```python
from build123d import *

# Parameters (mm, degrees)
F0_R      = 55.0458583504
F1_DEPTH  = 4
F2_R      = 41.0058886934
F3_DEPTH  = 1
F4_R      = 11.9318178019
F5_DEPTH  = 2
F6_R      = 8.7944266384
F7_DEPTH  = 1
F8_R      = 5.553220806
F9_DEPTH  = 1
F11_DEPTH = 2
F13_DEPTH = 2


with BuildPart() as f1:
    # F0 (on Top) → F1 (new body)
    with BuildSketch(Plane.XY):
        Circle(F0_R)
    extrude(amount=F1_DEPTH)

    # F2 (on face) → F3 (join)
    with BuildSketch(Plane.XY.offset(4)):
        Circle(F2_R)
    extrude(amount=F3_DEPTH)

    # F4 (on face) → F5 (cut)
    with BuildSketch(Plane.XY.offset(5)):
        Circle(F4_R)
    extrude(amount=-F5_DEPTH, mode=Mode.SUBTRACT)

    # F6 (on face) → F7 (join)
    with BuildSketch(Plane.XY.offset(3)):
        Circle(F6_R)
    extrude(amount=F7_DEPTH)

    # F8 (on face) → F9 (join)
    with BuildSketch(Plane.XY.offset(4)):
        Circle(F8_R)
    extrude(amount=F9_DEPTH)

    # F10 (on face) → F11 (cut)
    with BuildSketch(Plane.XY.offset(5)):
        with BuildLine():
            Line((-11.5631810567, 2.9429780682), (-40.9001441028, 2.9429780682))
            ThreePointArc((-40.9001441028, 2.9429780682), (-41.0058886934, 0), (-40.9001441028, -2.9429780682))
            Line((-40.9001441028, -2.9429780682), (-11.5631810567, -2.9429780682))
            ThreePointArc((-11.5631810567, -2.9429780682), (-11.9318178019, 0), (-11.5631810567, 2.9429780682))
        make_face()
    extrude(amount=-F11_DEPTH, mode=Mode.SUBTRACT)

    # F12 (on face) → F13 (cut)
    with BuildSketch(Plane.XY.offset(5)):
        with BuildLine():
            Line((40.8989598294, 2.959390547), (11.5589914633, 2.959390547))
            ThreePointArc((11.5589914633, 2.959390547), (11.9318147961, 0.0084693883), (11.5631810567, -2.9429780682))
            Line((11.5631810567, -2.9429780682), (40.9001441028, -2.9429780682))
            ThreePointArc((40.9001441028, -2.9429780682), (41.005887868, 0.008227575), (40.8989598294, 2.959390547))
        make_face()
    extrude(amount=-F13_DEPTH, mode=Mode.SUBTRACT)


solid = f1.part
```
Can you work these out from the model? Positions are in its coordinate system, mm. A direction names the side the tool comes from. Give positions to 0.01 mm unless a question says otherwise; leave off trailing zeros. Order: outer loops, then holes, each group sorted by start corner. A loop starts at its lowest first (then second) coordinate and runs counter-clockwise, first axis right, second up. Notation, with made-up numbers: (52.5, 0) - (106.5, 0) arc R29 cw to (106.5, 33) - close; hole circle Ø2 at (69, 37). An arc over 180 degrees is marked (long way). Use a Markdown table: item, result. Add a question column.
Q1. If we mould it in two halves opening along X, with no side actions, what happens to faces 4 (the flat face through (0, 0, 5)), 5 (the flat face through (0, -6, 4)), 6 (the cylindrical face through (-0.22, -11.93, 4.01)), 7 (the cylindrical face through (0.852, 40.997, 4.493))? For each: released by +X, released by -X, zero draft, split by the parting line, or undercut.
Q2. On a 3-axis mill with a long thin cutter (end or side, diameter ignored), from which of +Z, -Z, +X, -X, +Y, -Y can I reach the whole of each face in a straight line? I mean faces 1 (the flat face through (-1, -22, 5)), 2 (the cylindrical face through (-0.86, -40.997, 4.493)), 3 (the cylindrical face through (-1.2, -5.42, 4.49)). Say none if no direction works.
Q3. If we section it at A-A on y = 0: Write out the boundary of the cut face in (x, z).
Q4. If we section it at C-C on z = 1.9: Write out the boundary of the cut face in (x, y).
Q5. If we section it at B-B on x = 0: Write out the boundary of the cut face in (y, z).
Q6. I'm going to push flat-ended pins straight in: pin 1 (1.5 mm diameter, centred on y = -9.5, z = 2.5, fed in from -X); pin 2 (2 mm diameter, centred on x = 19.5, z = 4.5, fed in from -Y); pin 3 (1.6 mm diameter, centred on x = 23.5, z = 4, fed in from +Y). Where does each tip first touch, or does it pass through?
Q7. If we section it at D-D on x = 28: Write out the boundary of the cut face in (y, z), plus the area to 3 significant figures.
Q8. Please list where these lines run through material, in increasing order: line 1 along Y through (x, z) = (0, 3.6); line 2 along Y through (x, z) = (-5, 3.05); line 3 along Y through (x, z) = (1, 1.5).
Answers follow:
| question | item | result |
|---|---|---|
| 1 | face 4 | zero draft |
| 1 | face 5 | undercut |
| 1 | face 6 | undercut |
| 1 | face 7 | split by the parting line |
| 2 | face 1 | +Z, +X, -X, +Y, -Y |
| 2 | face 2 | +Z, -Y |
| 2 | face 3 | +Z |
| 3 | outline | (-55.05, 0) - (55.05, 0) - (55.05, 4) - (41.01, 4) - (41.01, 3) - (8.79, 3) - (8.79, 4) - (5.55, 4) - (5.55, 5) - (-5.55, 5) - (-5.55, 4) - (-8.79, 4) - (-8.79, 3) - (-41.01, 3) - (-41.01, 4) - (-55.05, 4) - close |
| 4 | outline | circle Ø110.09 at (0, 0) |
| 5 | outline | (-55.05, 0) - (55.05, 0) - (55.05, 4) - (41.01, 4) - (41.01, 5) - (11.93, 5) - (11.93, 3) - (8.79, 3) - (8.79, 4) - (5.55, 4) - (5.55, 5) - (-5.55, 5) - (-5.55, 4) - (-8.79, 4) - (-8.79, 3) - (-11.93, 3) - (-11.93, 5) - (-41.01, 5) - (-41.01, 4) - (-55.05, 4) - close |
| 6 | pin 1 | stops at x = -54.35 |
| 6 | pin 2 | stops at y = -51.8 |
| 6 | pin 3 | stops at y = 50.15 |
| 7 | outline | (-47.39, 0) - (47.39, 0) - (47.39, 4) - (29.96, 4) - (29.96, 5) - (2.96, 5) - (2.96, 3) - (-2.94, 3) - (-2.94, 5) - (-29.96, 5) - (-29.96, 4) - (-47.39, 4) - close |
| 7 | area | 427 mm^2 |
| 8 | line 1 | y = -55.05 to -11.93, -8.79 to 8.79, 11.93 to 55.05 |
| 8 | line 2 | y = -54.82 to -10.83, -7.23 to 7.23, 10.83 to 54.82 |
| 8 | line 3 | y = -55.04 to 55.04 |
